Autodesk Inventor part; units mm, degrees
ref_plane "YZ Plane" through (0, 0, 0) normal (1, 0, 0) x (0, 1, 0)
ref_plane "XZ Plane" through (0, 0, 0) normal (0, 1, 0) x (-1, 0, 0)
ref_plane "XY Plane" through (0, 0, 0) normal (0, 0, 1) x (1, 0, 0)
sketch "Sketch1" plane through (0, 0, 0) normal (0, 1, 0) x (-1, 0, 0)
  circle A0 centre (0, 0) radius 17.5
  circle A1 centre (0, 0) radius 22
  dimension "d0" = 35
  dimension "d1" = 44
extrude "Extrusion1" add sketch "Sketch1" along normal blind 5
sketch "Sketch2" plane through (0, 5, 0) normal (0, 1, 0) x (1, 0, 0)
  circle A0 centre (0, 0) radius 22
  circle A1 centre (0, 0) radius 17.5
  circle A2 centre (0, 0) radius 19
  circle A3 centre (0, 0) radius 20.5
  dimension "d4" = 38
  dimension "d5" = 41
extrude "Extrusion2" cut sketch "Sketch2" against normal blind 0.5 contours A3
sketch "Sketch3" plane through (0, 0, 0) normal (0, -1, 0) x (1, 0, 0)
  circle A0 centre (0, 0) radius 19
  circle A1 centre (0, 0) radius 20.5
extrude "Extrusion3" cut sketch "Sketch3" against normal blind 0.5
properties part number "bearing_35_44_5" material "Stainless Steel"
The model under review builds one solid part; all positions refer to its coordinate system, in mm. A direction names the side the tool comes from. Coordinates: 2 decimals unless noted, no trailing zeros. Write each loop counter-clockwise with the first axis right and the second up, starting at its lowest first coordinate (ties: lowest second). Pieces come first, ordered by that corner, then holes. Notation, with made-up numbers: (27, 44.5) -> (35, 44.5) arc R7 cw to (35, 56.5) -> close; hole circle Ø1 at (31.25, 46). An arc over 180 degrees is marked (long way). One line per item, written item: value. Start each with the question number.
Q1. For faces 1 (the face through (8.767, 4.754, 16.856)), 2 (the face through (8.767, 0.246, -16.856)), 3 (the face through (4.769, 2.465, 21.477)), list the 3-axis set-ups (+Z, -Z, +X, -X, +Y, -Y) from which the entire face can be reached by the end or side of a thin tool; tool diameter is ignored.
Q2. The part is to be moulded in two halves that separate along Y. For faces 4 (the face through (-15, 0, -15)), 5 (the face through (-15, 5, -15)), 6 (the face through (13.887, 2.465, 10.648)), say which applies: +Y half, -Y half, draft (parallel to the pull), parting line (faces both ways), or undercut.
Q3. Add section B-B, the plane x = 0. Give the boundary of the cut face in (y, z), then the cut area to 3 significant figures.
Q4. Clearance check with flat-ended pins moving along their axes: P1, Ø1, axis at x = 7.5, y = 3, coming from the -Z side; P2, Ø1, axis at y = 4, z = 12.5, coming from the +X side; P3, Ø2, axis at x = 5.5, y = 3.5, coming from the +Z side. State where each tip first meets the part, or that it passes through.
Q5. Add section C-C, the plane y = 2.35. Give the boundary of the cut face in (x, z), then the cut area to 3 significant figures.
Q6. Add section A-A, the plane z = 0. Give the boundary of the cut face in (x, y).
Q7. To check wall thickness, follow probe 1 along Z at (x, y) = (0, 4.65); probe 2 along Z at (x, y) = (-0.5, 3.35); probe 3 along Z at (x, y) = (7.5, 3.1). State the ranges of each line that lie inside material, in increasing order.
Response:
1. face 1: +Y
1. face 2: -Y
1. face 3: +Y, -Y
2. face 4: -Y half
2. face 5: +Y half
2. face 6: draft
3. outline: (0, -22) -> (5, -22) -> (5, -20.5) -> (4.5, -20.5) -> (4.5, -19) -> (5, -19) -> (5, -17.5) -> (0, -17.5) -> (0, -19) -> (0.5, -19) -> (0.5, -20.5) -> (0, -20.5) -> close; (0, 17.5) -> (5, 17.5) -> (5, 19) -> (4.5, 19) -> (4.5, 20.5) -> (5, 20.5) -> (5, 22) -> (0, 22) -> (0, 20.5) -> (0.5, 20.5) -> (0.5, 19) -> (0, 19) -> close
3. area: 42.0 mm²
4. P1: z = -20.86
4. P2: x = 18.44
4. P3: z = 21.53
5. outline: circle Ø44 at (0, 0); hole circle Ø35 at (0, 0)
5. area: 558 mm²
6. outline: (-22, 0) -> (-20.5, 0) -> (-20.5, 0.5) -> (-19, 0.5) -> (-19, 0) -> (-17.5, 0) -> (-17.5, 5) -> (-19, 5) -> (-19, 4.5) -> (-20.5, 4.5) -> (-20.5, 5) -> (-22, 5) -> close; (17.5, 0) -> (19, 0) -> (19, 0.5) -> (20.5, 0.5) -> (20.5, 0) -> (22, 0) -> (22, 5) -> (20.5, 5) -> (20.5, 4.5) -> (19, 4.5) -> (19, 5) -> (17.5, 5) -> close
7. probe 1: -22 to -20.5, -19 to -17.5, 17.5 to 19, 20.5 to 22
7. probe 2: -21.99 to -17.49, 17.49 to 21.99
7. probe 3: -20.68 to -15.81, 15.81 to 20.68
